Autodesk Inventor part; units mm, degrees
ref_plane "YZ Plane" through (0, 0, 0) normal (1, 0, 0) x (0, 1, 0)
ref_plane "XZ Plane" through (0, 0, 0) normal (0, 1, 0) x (-1, 0, 0)
ref_plane "XY Plane" through (0, 0, 0) normal (0, 0, 1) x (1, 0, 0)
sketch "Sketch1" plane through (0, 0, 0) normal (0, 0, 1) x (1, 0, 0)
  circle A0 centre (0, 0) radius 5.08
  arc A1 (0, 16) -> (0, -16) centre (0, 0) ccw
  line L0 (0, 16) -> (99.4033, 16)
  line L1 (99.4033, 16) -> (99.4033, -16)
  line L2 (99.4033, -16) -> (0, -16)
  line L3 (0, -16) -> (0, 16) construction
  line L4 (39.8634, 25) -> (99.4033, 25)
  line L5 (99.4033, 25) -> (99.4033, -25)
  line L6 (99.4033, -25) -> (39.8634, -25)
  line L7 (39.8634, -25) -> (39.8634, 25)
  arc A2 (39.8634, -25) -> (0, -16) centre (0, -108.7828) ccw
  arc A3 (0, 16) -> (39.8634, 25) centre (0, 108.7828) ccw
  circle A4 centre (50.0625, 0) radius 2
  circle A5 centre (90.0625, 0) radius 2
  line L8 (-16, 0) -> (99.4033, 0) construction
  point P0 (39.8634, 0)
  dimension "d1" = 10.16
  dimension "d3" = 50
  dimension "d4" = 59.5399
  dimension "d12" = 4
  dimension "d13" = 40
  dimension "d14" = 50.0625
  dimension "d15" = 9.3408
  dimension "d44" = 16
extrude "Extrusion1" add sketch "Sketch1" along normal blind 5
ref_plane "Work Plane1" through (39.8634, 0, 0) normal (0, -1, 0) x (1, 0, 0)
sketch "Sketch4" plane through (0, 0, 5) normal (0, 0, 1) x (1, 0, 0)
  arc A0 (15, 6) -> (47.3064, 15.8305) centre (15, 64.0002) ccw
  arc A1 (15, 4) -> (48.4204, 14.1695) centre (15, 64.0002) ccw
  circle A2 centre (47.8634, 15) radius 1
  circle A3 centre (15, 5) radius 1
  arc A4 (0, 16) -> (39.8634, 25) centre (0, 108.7828) ccw
  line L0 (99.4033, 25) -> (39.8634, 25)
  line L1 (122.484, 0) -> (-39.0807, 0)
  line L2 (15, 4) -> (47.8634, 4) construction
  point P0 (0, 0)
  dimension "d16" = 2
  dimension "d17" = 10
  dimension "d18" = 8
  dimension "d19" = 15
  dimension "d20" = 5
extrude "Extrusion3" cut sketch "Sketch4" against normal through all
mirror "Mirror1" about plane through (39.8634, 0, 0) normal (0, -1, 0) of "Extrusion3"
sketch "Sketch5" plane through (0, 0, 0) normal (0, 0, -1) x (-1, 0, 0)
  arc A0 (-15, -4) -> (-48.4204, -14.1695) centre (-15, -64.0002) ccw
  arc A1 (-15, -6) -> (-15, -4) centre (-15, -5) ccw
  arc A2 (-15, -6) -> (-47.3064, -15.8305) centre (-15, -64.0002) ccw
  arc A3 (-48.4204, -14.1695) -> (-47.3064, -15.8305) centre (-47.8634, -15) ccw
  arc A4 (-47.3064, 15.8305) -> (-15, 6) centre (-15, 64.0002) ccw
  arc A5 (-15, 4) -> (-15, 6) centre (-15, 5) ccw
  arc A6 (-48.4204, 14.1695) -> (-15, 4) centre (-15, 64.0002) ccw
  arc A7 (-47.3064, 15.8305) -> (-48.4204, 14.1695) centre (-47.8634, 15) ccw
  arc A8 (0, -16) -> (0, 16) centre (0, 0) ccw
  arc A9 (-39.8634, 25) -> (0, 16) centre (0, 108.7828) ccw
  line L0 (-99.4033, 25) -> (-39.8634, 25)
  line L1 (-99.4033, -25) -> (-99.4033, 25)
  line L2 (-39.8634, -25) -> (-99.4033, -25)
  arc A10 (0, -16) -> (-39.8634, -25) centre (0, -108.7828) ccw
  circle A11 centre (-50.0625, 0) radius 2
  circle A12 centre (-90.0625, 0) radius 2
  circle A13 centre (0, 0) radius 5.08
  line L3 (-39.8634, 25) -> (-47.8634, 25)
  line L4 (-47.8634, 25) -> (-47.8634, 22.5)
  line L5 (-47.8634, 22.5) -> (-39.8634, 22.5)
  line L6 (-39.8634, 22.5) -> (-39.8634, 25)
  dimension "d23" = 8
  dimension "d24" = 2.5
extrude "Extrusion4" add sketch "Sketch5" along normal blind 8 contours L6 L5 L4 L0
sketch "Sketch6" plane through (39.8634, 25, 5) normal (0, 1, 0) x (1, 0, 0)
  line L0 (59.5399, 5) -> (8, 5)
  line L1 (8, 5) -> (8, 13)
  line L2 (0, 13) -> (8, 13)
  line L3 (0, 5) -> (0, 13)
  line L4 (0, 5) -> (0, 0)
  line L5 (59.5399, 0) -> (0, 0)
  line L6 (59.5399, 5) -> (59.5399, 0)
  circle A0 centre (4, 9) radius 2
  line L7 (4, 13) -> (4, 9) construction
  point P0 (-39.8634, 5)
  dimension "d27" = 4
  dimension "d28" = 4
extrude "Extrusion5" cut sketch "Sketch6" against normal up to next contours A0
mirror "Mirror2" about plane through (39.8634, 0, 0) normal (0, -1, 0) of "Extrusion4", "Extrusion5"
sketch "Sketch7" plane through (0, 0, 0) normal (0, 0, -1) x (-1, 0, 0)
  circle A0 centre (0, 0) radius 5.08
  circle A1 centre (-90.0625, 0) radius 2
  circle A2 centre (-50.0625, 0) radius 2
  arc A3 (-47.3064, 15.8305) -> (-15, 6) centre (-15, 64.0002) ccw
  arc A4 (-15, 4) -> (-15, 6) centre (-15, 5) ccw
  arc A5 (-48.4204, 14.1695) -> (-15, 4) centre (-15, 64.0002) ccw
  arc A6 (-47.3064, 15.8305) -> (-48.4204, 14.1695) centre (-47.8634, 15) ccw
  arc A7 (-15, -4) -> (-48.4204, -14.1695) centre (-15, -64.0002) ccw
  arc A8 (-15, -6) -> (-15, -4) centre (-15, -5) ccw
  arc A9 (-15, -6) -> (-47.3064, -15.8305) centre (-15, -64.0002) ccw
  arc A10 (-48.4204, -14.1695) -> (-47.3064, -15.8305) centre (-47.8634, -15) ccw
  line L0 (-47.8634, -25) -> (-47.8634, -22.5)
  line L1 (-47.8634, -22.5) -> (-39.8634, -22.5)
  line L2 (-39.8634, -22.5) -> (-39.8634, -25)
  arc A11 (0, -16) -> (-39.8634, -25) centre (0, -108.7828) ccw
  arc A12 (0, -16) -> (0, 16) centre (0, 0) ccw
  arc A13 (-39.8634, 25) -> (0, 16) centre (0, 108.7828) ccw
  line L3 (-39.8634, 25) -> (-39.8634, 22.5)
  line L4 (-39.8634, 22.5) -> (-47.8634, 22.5)
  line L5 (-47.8634, 22.5) -> (-47.8634, 25)
  line L6 (-99.4033, 25) -> (-47.8634, 25)
  line L7 (-99.4033, -25) -> (-99.4033, 25)
  line L8 (-47.8634, -25) -> (-99.4033, -25)
  circle A14 centre (-70.0625, 21) radius 10
  arc A15 (-65.0249, 29.6384) -> (-47.8634, 25) centre (-47.8634, 59.0667) ccw
  line L9 (-99.4033, 25) -> (-47.8634, 25)
  line L10 (39.0807, 0) -> (-122.484, 0)
  line L11 (-70.0625, -25) -> (-70.0625, 21) construction
  line L12 (-90.0625, 0) -> (-50.0625, 0) construction
  line L13 (0, 16) -> (-99.4033, 16) construction
  arc A16 (-99.4033, 16) -> (-78.1686, 26.8559) centre (-99.4033, 42.1961) ccw
  point P0 (-92.2616, 25)
  point P1 (-75.1001, 29.6384)
  point P2 (-70.0625, 0)
  point P3 (-60.8973, 25)
  point P4 (-79.2277, 25)
  point P5 (-79.6415, 25)
  dimension "d31" = 20
  dimension "d32" = 21
extrude "Extrusion6" add sketch "Sketch7" against normal up to surface (5 mm away) contours L6 A14 A15 | L6 A14 | A16 A14 L6 picked at (-67.4658, 26.7505)
sketch "Sketch8" plane through (0, 0, 0) normal (0, 0, -1) x (-1, 0, 0)
  circle A0 centre (0, 0) radius 5.08
  circle A1 centre (-90.0625, 0) radius 2
  circle A2 centre (-50.0625, 0) radius 2
  arc A3 (-47.3064, 15.8305) -> (-15, 6) centre (-15, 64.0002) ccw
  arc A4 (-15, 4) -> (-15, 6) centre (-15, 5) ccw
  arc A5 (-48.4204, 14.1695) -> (-15, 4) centre (-15, 64.0002) ccw
  arc A6 (-47.3064, 15.8305) -> (-48.4204, 14.1695) centre (-47.8634, 15) ccw
  arc A7 (-15, -4) -> (-48.4204, -14.1695) centre (-15, -64.0002) ccw
  arc A8 (-15, -6) -> (-15, -4) centre (-15, -5) ccw
  arc A9 (-15, -6) -> (-47.3064, -15.8305) centre (-15, -64.0002) ccw
  arc A10 (-48.4204, -14.1695) -> (-47.3064, -15.8305) centre (-47.8634, -15) ccw
  line L0 (-47.8634, -25) -> (-47.8634, -22.5)
  line L1 (-47.8634, -22.5) -> (-39.8634, -22.5)
  line L2 (-39.8634, -22.5) -> (-39.8634, -25)
  arc A11 (0, -16) -> (-39.8634, -25) centre (0, -108.7828) ccw
  arc A12 (0, -16) -> (0, 16) centre (0, 0) ccw
  arc A13 (-39.8634, 25) -> (0, 16) centre (0, 108.7828) ccw
  line L3 (-39.8634, 25) -> (-39.8634, 22.5)
  line L4 (-39.8634, 22.5) -> (-47.8634, 22.5)
  line L5 (-47.8634, 22.5) -> (-47.8634, 25)
  arc A14 (-65.0249, 29.6384) -> (-47.8634, 25) centre (-47.8634, 59.0667) ccw
  arc A15 (-65.0249, 29.6384) -> (-78.1686, 26.8559) centre (-70.0625, 21) ccw
  line L6 (-99.4033, 25) -> (-79.6415, 25)
  line L7 (-99.4033, -25) -> (-99.4033, 25)
  line L8 (-47.8634, -25) -> (-99.4033, -25)
  circle A16 centre (-70.0625, 21) radius 6.5
  arc A17 (-79.6415, 25) -> (-78.1686, 26.8559) centre (-99.4033, 42.1961) ccw
  dimension "d35" = 13
extrude "Extrusion7" add sketch "Sketch8" along normal blind 5 contours A16
sketch "Sketch9" plane through (70.0625, 21, -5) normal (0, 0, -1) x (-1, 0, 0)
  circle A0 centre (0, 0) radius 3.5
  circle A1 centre (0, 0) radius 6.5
  point P0 (70.0625, -21)
  dimension "d38" = 7
extrude "Extrusion8" add sketch "Sketch9" along normal blind 10 contours A0
fillet "Fillet1" radius 2 1 edges at (73.5625, 21, -15)
extrude "Extrusion9" cut sketch "Sketch7" against normal through all contours L7 L6 A16
mirror "Mirror3" about plane through (39.8634, 0, 0) normal (0, -1, 0) of "Extrusion6", "Extrusion7", "Extrusion8", "Fillet1", "Extrusion9"
sketch "Sketch10" plane through (0, 0, 5) normal (0, 0, 1) x (1, 0, 0)
  arc A0 (48.4204, -14.1695) -> (15, -4) centre (15, -64.0002) ccw
  arc A1 (47.3064, -15.8305) -> (48.4204, -14.1695) centre (47.8634, -15) ccw
  arc A2 (47.3064, -15.8305) -> (15, -6) centre (15, -64.0002) ccw
  arc A3 (15, -4) -> (15, -6) centre (15, -5) ccw
  arc A4 (15, 6) -> (47.3064, 15.8305) centre (15, 64.0002) ccw
  arc A5 (48.4204, 14.1695) -> (47.3064, 15.8305) centre (47.8634, 15) ccw
  arc A6 (15, 4) -> (48.4204, 14.1695) centre (15, 64.0002) ccw
  arc A7 (15, 6) -> (15, 4) centre (15, 5) ccw
  arc A8 (99.4033, -16) -> (78.1686, -26.8559) centre (99.4033, -42.1961) ccw
  line L0 (99.4033, -16) -> (99.4033, 16)
  arc A9 (78.1686, 26.8559) -> (99.4033, 16) centre (99.4033, 42.1961) ccw
  line L1 (47.8634, 25) -> (39.8634, 25)
  arc A10 (78.1686, 26.8559) -> (65.0249, 29.6384) centre (70.0625, 21) ccw
  arc A11 (47.8634, 25) -> (65.0249, 29.6384) centre (47.8634, 59.0667) ccw
  arc A12 (0, 16) -> (39.8634, 25) centre (0, 108.7828) ccw
  arc A13 (0, 16) -> (0, -16) centre (0, 0) ccw
  arc A14 (39.8634, -25) -> (0, -16) centre (0, -108.7828) ccw
  line L2 (39.8634, -25) -> (47.8634, -25)
  arc A15 (65.0249, -29.6384) -> (47.8634, -25) centre (47.8634, -59.0667) ccw
  arc A16 (65.0249, -29.6384) -> (78.1686, -26.8559) centre (70.0625, -21) ccw
  circle A17 centre (50.0625, 0) radius 2
  circle A18 centre (90.0625, 0) radius 2
  circle A19 centre (0, 0) radius 5.08
  circle A20 centre (50.0625, 0) radius 4
  circle A21 centre (90.0625, 0) radius 4
  dimension "d45" = 8
extrude "Extrusion10" cut sketch "Sketch10" against normal blind 2.5 contours A20 | A21
sketch "Sketch11" plane through (0, 0, 5) normal (0, 0, 1) x (1, 0, 0)
  circle A0 centre (0, 0) radius 7.235
  dimension "d48" = 14.47
extrude "Extrusion11" cut sketch "Sketch11" against normal blind 2
sketch "Sketch12" plane through (0, 0, 0) normal (0, 0, -1) x (-1, 0, 0)
  circle A0 centre (-70.0625, 21) radius 1.5
  circle A1 centre (-70.0625, 21) radius 10
  circle A2 centre (-90.0625, 0) radius 2
  circle A3 centre (-90.0625, 0) radius 10
  circle A4 centre (-70.0625, -21) radius 1.5
  circle A5 centre (-70.0625, -21) radius 10
  circle A6 centre (-90.0625, 0) radius 2
  arc A7 (-79.7352, -23.5375) -> (-93.0685, -9.5375) centre (-99.0806, -28.6125) ccw
  arc A8 (-93.0685, 9.5375) -> (-79.7352, 23.5375) centre (-99.0806, 28.6125) ccw
  arc A9 (-78.1686, -26.8559) -> (-99.4033, -16) centre (-99.4033, -42.1961) ccw
  arc A10 (-78.1686, -26.8559) -> (-65.0249, -29.6384) centre (-70.0625, -21) ccw
  arc A11 (-47.8634, -25) -> (-65.0249, -29.6384) centre (-47.8634, -59.0667) ccw
  line L0 (-47.8634, -25) -> (-47.8634, -22.5)
  line L1 (-47.8634, -22.5) -> (-39.8634, -22.5)
  line L2 (-39.8634, -22.5) -> (-39.8634, -25)
  arc A12 (0, -16) -> (-39.8634, -25) centre (0, -108.7828) ccw
  arc A13 (0, -16) -> (0, 16) centre (0, 0) ccw
  arc A14 (-39.8634, 25) -> (0, 16) centre (0, 108.7828) ccw
  line L3 (-39.8634, 25) -> (-39.8634, 22.5)
  line L4 (-39.8634, 22.5) -> (-47.8634, 22.5)
  line L5 (-47.8634, 22.5) -> (-47.8634, 25)
  arc A15 (-65.0249, 29.6384) -> (-47.8634, 25) centre (-47.8634, 59.0667) ccw
  arc A16 (-65.0249, 29.6384) -> (-78.1686, 26.8559) centre (-70.0625, 21) ccw
  arc A17 (-99.4033, 16) -> (-78.1686, 26.8559) centre (-99.4033, 42.1961) ccw
  line L6 (-99.4033, -16) -> (-99.4033, 16)
  circle A18 centre (-70.0625, -21) radius 6.5
  circle A19 centre (-70.0625, 21) radius 6.5
  circle A20 centre (0, 0) radius 5.08
  circle A21 centre (-90.0625, 0) radius 2
  circle A22 centre (-50.0625, 0) radius 2
  arc A23 (-47.3064, 15.8305) -> (-15, 6) centre (-15, 64.0002) ccw
  arc A24 (-15, 4) -> (-15, 6) centre (-15, 5) ccw
  arc A25 (-48.4204, 14.1695) -> (-15, 4) centre (-15, 64.0002) ccw
  arc A26 (-47.3064, 15.8305) -> (-48.4204, 14.1695) centre (-47.8634, 15) ccw
  arc A27 (-15, -4) -> (-48.4204, -14.1695) centre (-15, -64.0002) ccw
  arc A28 (-15, -6) -> (-15, -4) centre (-15, -5) ccw
  arc A29 (-15, -6) -> (-47.3064, -15.8305) centre (-15, -64.0002) ccw
  arc A30 (-48.4204, -14.1695) -> (-47.3064, -15.8305) centre (-47.8634, -15) ccw
  point P0 (-99.4033, -3.5706)
  point P1 (-99.4033, 3.5706)
  dimension "d54" = 20
  dimension "d56" = 20
  dimension "d55" = 20
  dimension "d57" = 4
  dimension "d58" = 20
  dimension "d59" = 20
extrude "Extrusion12" cut sketch "Sketch12" against normal blind 10 contours A8 A3 L6 A17 A1 | A7 A5 A9 L6 A3
extrude "Extrusion13" add sketch "Sketch12" against normal up to surface (5 mm away) contours L6 A3 picked at (-99.5984, 0.4047)
chamfer "Chamfer1" distance 2 angle 45 5 edges at (20.4334, 18.278, 5) (-16, 0, 5) (20.4334, -18.278, 5) (43.8634, 25, 5) (43.8634, -25, 5)
equation "\"d59\" = d58"
properties part number "Bearing_Arm_3DPrint"
Part model, mm, in its own coordinate system. A direction names the side the tool comes from. Give positions to 0.01 mm unless a question says otherwise; leave off trailing zeros.
1) Which spindle directions (+Z, -Z, +X, -X, +Y, -Y) get a long thin tool onto all of the face, cutting with end or side? Do faces 1 (the face through (44, -25, -1)), 2 (the face through (72.64, -23.37, -8.94)), 3 (the face through (44, 24, 4)), 4 (the face through (14, -5, 3)), 5 (the face through (44, -24, -8)). Say none if no direction does.
Resolved:
face 1: +Z, -Z, -X, -Y
face 2: -Z
face 3: +Z, -X, +Y
face 4: +Z, -Z
face 5: -Z, -X, +Y, -Y
2) Two-plate mould, pull along Y, no slides. Class faces 6 (the face through (56.874, 26.213, 1.479)), 7 (the face through (-0.661, -5.037, 1.479)), 8 (the face through (45.71, 23.77, -3.23)): released by +Y, released by -Y, zero draft, split by the parting line, or undercut.
Resolved:
face 6: released by +Y
face 7: undercut
face 8: zero draft
3) Probe L1, parallel to Y at x = 45.5, z = -2.5; L2, parallel to Y at x = 19.5, z = 1; L3, parallel to X at y = 23.6, z = -4. List the from-to ranges inside material, lowest first.
Resolved:
L1: y = -25 to -22.5, 22.5 to 25
L2: y = -18.07 to -6.17, -4.17 to 4.17, 6.17 to 18.07
L3: x = 39.86 to 41.86, 45.86 to 47.86, 64.11 to 76.02
4) Pin check, flat tips, straight feed: pin 1 (2.5 mm diameter, centred on x = 45.5, z = -2.5, fed in from -Y); pin 2 (4.5 mm diameter, centred on x = 50.06, y = 0, fed in from +Z); pin 3 (0.8 mm diameter, centred on x = 45, y = -23.5, fed in from -Z); pin 4 (6 mm diameter, centred on x = 0, y = 0, fed in from +Z). Stop position of each tip, or through.
Resolved:
pin 1: stops at y = -25
pin 2: stops at z = 2.5
pin 3: stops at z = -8
pin 4: passes through
5) Cut at A-A on y = 0. State how many separate pieces and enclosed holes the cut face has, then the cut area to 3 significant figures.
Resolved:
separate pieces: 4
enclosed holes: 0
area: 457 mm2
